For this review, take the finished solid that the model builds, in its own axes (mm). Face numbers are marked on the shaded views. Coordinates: 2 decimals unless noted, no trailing zeros. Loops run counter-clockwise (first coordinate to the right, second up) from the corner with the lowest first, then second, coordinate; pieces in that order, holes last. Notation, with made-up numbers: (52, 29) -> (87, 29) arc R4 ccw to (87, 34) -> close; hole circle Ø3 at (-25.5, 74). An arc over 180 degrees is marked (long way). Answer in a Markdown table with one row per item.
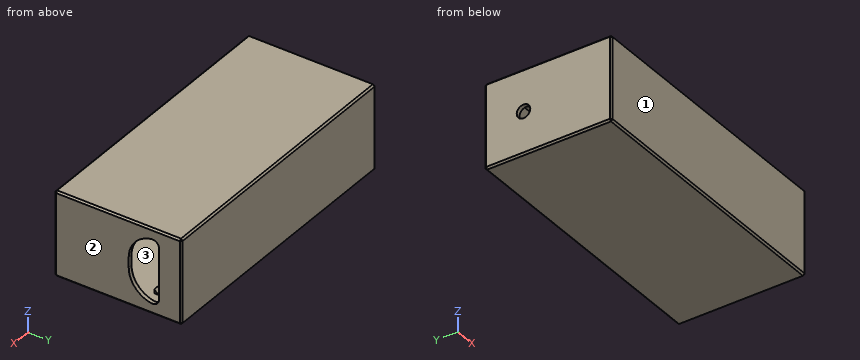
from build123d import *

# Parameters (mm, degrees)
SKETCH1_W           = 82.5
SKETCH1_H           = 25
SKETCH1_W_2         = 80.1
SKETCH1_H_2         = 22.6
BOSS_EXTRUDE1_DEPTH = 23.2
SKETCH1_2_W         = 82.5
SKETCH1_2_H         = 25
SKETCH1_2_W_2       = 80.1
SKETCH1_2_H_2       = 22.6
BOSS_EXTRUDE2_DEPTH = 2
SKETCH2_W           = 2.5
SKETCH2_H           = 5.55
BOSS_EXTRUDE3_DEPTH = 5
SKETCH8_W           = 82.5
SKETCH8_H           = 25
SKETCH8_W_2         = 80.1
SKETCH8_H_2         = 22.6
BOSS_EXTRUDE4_DEPTH = 11.2
SKETCH10_W          = 82.5
SKETCH10_H          = 25
BOSS_EXTRUDE6_DEPTH = 1.2
SKETCH11_W          = 19
SKETCH11_H          = 9
CUT_EXTRUDE1_DEPTH  = 1.2
FILLET1_R           = 8
FILLET2_R           = 2
CHAMFER1_SIZE       = 0.5
CHAMFER2_SIZE       = 2
SKETCH12_R          = 2
CUT_EXTRUDE2_DEPTH  = 1.2


with BuildPart() as part:
    # Sketch1 → Boss-Extrude1 (new body)
    with BuildSketch(Plane(origin=(0, 0, 0), x_dir=(1, 0, 0), z_dir=(0, 1, 0))):
        Rectangle(SKETCH1_W, SKETCH1_H)
        Rectangle(SKETCH1_W_2, SKETCH1_H_2, mode=Mode.SUBTRACT)
    extrude(amount=BOSS_EXTRUDE1_DEPTH)

    # Sketch1_2 → Boss-Extrude2 (add)
    # profile 1 of 2: a face of its own
    with BuildSketch(Plane(origin=(0, 0, 0), x_dir=(1, 0, 0), z_dir=(0, 1, 0))):
        Rectangle(SKETCH1_2_W, SKETCH1_2_H)
        Rectangle(SKETCH1_2_W_2, SKETCH1_2_H_2, mode=Mode.SUBTRACT)
    # profile 2 of 2: a face of its own
    with BuildSketch(Plane(origin=(0, 0, 0), x_dir=(1, 0, 0), z_dir=(0, 1, 0))):
        Rectangle(SKETCH1_2_W_2, SKETCH1_2_H_2)
    extrude(amount=-BOSS_EXTRUDE2_DEPTH)

    # Sketch2 → Boss-Extrude3 (add)
    with BuildSketch(Plane(origin=(0, 0, 0), x_dir=(1, 0, 0), z_dir=(0, 1, 0))):
        with Locations((-38.8, 8.525)):
            Rectangle(SKETCH2_W, SKETCH2_H)
        with Locations((-38.8, -8.525)):
            Rectangle(SKETCH2_W, SKETCH2_H)
        with Locations((38.8, -8.525)):
            Rectangle(SKETCH2_W, SKETCH2_H)
        with Locations((38.8, 8.525)):
            Rectangle(SKETCH2_W, SKETCH2_H)
    extrude(amount=BOSS_EXTRUDE3_DEPTH)

    # Sweep2: sweep along a path in Sketch3
    with BuildLine(Plane(origin=(0, 23.2, 0), x_dir=(1, 0, 0), z_dir=(0, 1, 0))) as sweep2_path:
        Line((-35, 11.3), (35, 11.3))
    # Sketch4 → Sweep2 (sweep)
    with BuildSketch(Plane(origin=(0, 0, 0), x_dir=(0, 0, -1), z_dir=(1, 0, 0))):
        Polygon((10.1, 23.2), (11.3, 24.4), (12.5, 24.4), (12.5, 23.2), align=None)
    sweep2 = sweep(path=sweep2_path.line)

    # Mirror1: Sweep2 across plane
    add(sweep2.mirror(Plane.XY))

    # Sketch8 → Boss-Extrude4 (add)
    with BuildSketch(Plane(origin=(0, 23.2, 0), x_dir=(1, 0, 0), z_dir=(0, 1, 0))):
        Rectangle(SKETCH8_W, SKETCH8_H)
        Rectangle(SKETCH8_W_2, SKETCH8_H_2, mode=Mode.SUBTRACT)
    extrude(amount=BOSS_EXTRUDE4_DEPTH)

    # Sketch10 → Boss-Extrude6 (add)
    with BuildSketch(Plane(origin=(0, 34.4, 0), x_dir=(1, 0, 0), z_dir=(0, 1, 0))):
        Rectangle(SKETCH10_W, SKETCH10_H)
    extrude(amount=BOSS_EXTRUDE6_DEPTH)

    # Sketch11 → Cut-Extrude1 (cut)
    with BuildSketch(Plane(origin=(41.25, 0, 0), x_dir=(0, 0, -1), z_dir=(1, 0, 0))):
        with Locations((0, 24.5)):
            Rectangle(SKETCH11_W, SKETCH11_H)
    extrude(amount=-CUT_EXTRUDE1_DEPTH, mode=Mode.SUBTRACT)

    # Fillet1
    fillet1_edges = [part.edges().sort_by_distance(p)[0] for p in [
        (40.65, 20, -9.5),
        (40.65, 20, 9.5),
    ]]
    fillet(fillet1_edges, radius=FILLET1_R)

    # Fillet2
    fillet2_edges = [part.edges().sort_by_distance(p)[0] for p in [
        (40.65, 29, 9.5),
        (40.65, 29, -9.5),
    ]]
    fillet(fillet2_edges, radius=FILLET2_R)

    # Chamfer1
    chamfer1_edges = [part.edges().sort_by_distance(p)[0] for p in [
        (0, 35.6, -12.5),
        (-41.25, 35.6, 0),
        (0, 35.6, 12.5),
        (41.25, 35.6, 0),
        (41.25, -2, 0),
        (0, -2, 12.5),
        (-41.25, -2, 0),
        (0, -2, -12.5),
        (-41.25, 16.8, -12.5),
        (41.25, 16.8, -12.5),
        (41.25, 16.8, 12.5),
        (-41.25, 16.8, 12.5),
    ]]
    chamfer(chamfer1_edges, length=CHAMFER1_SIZE)

    # Chamfer2
    chamfer2_edges = [part.edges().sort_by_distance(p)[0] for p in [
        (0, 34.4, -11.3),
        (-40.05, 34.4, 0),
        (0, 34.4, 11.3),
        (40.05, 34.4, 0),
    ]]
    chamfer(chamfer2_edges, length=CHAMFER2_SIZE)

    # Sketch12 → Cut-Extrude2 (cut)
    with BuildSketch(Plane.ZY.offset(41.25)):
        with Locations((0, 24)):
            Circle(SKETCH12_R)
    extrude(amount=-CUT_EXTRUDE2_DEPTH, mode=Mode.SUBTRACT)


solid = part.part
Item 1: Take a section at A-A, the plane z = 0. State the section outline as (x, y) points, and give its area (3 significant figures).
Worked answers:
| item | result |
|---|---|
| outline | (-41.25, -1.5) -> (-40.75, -2) -> (40.75, -2) -> (41.25, -1.5) -> (41.25, 20) -> (40.05, 20) -> (40.05, 0) -> (-40.05, 0) -> (-40.05, 22) -> (-41.25, 22) -> close; (-41.25, 26) -> (-40.05, 26) -> (-40.05, 32.4) -> (-38.05, 34.4) -> (38.05, 34.4) -> (40.05, 32.4) -> (40.05, 29) -> (41.25, 29) -> (41.25, 35.1) -> (40.75, 35.6) -> (-40.75, 35.6) -> (-41.25, 35.1) -> close |
| area | 334 mm² |
Item 2: Insertion check: pin 1 (1.3 mm diameter, centred on x = 41, z = 3.5, fed in from -Y). The pin has a flat end and moves straight along its axis. Give the tip position at first contact, or say it passes through.
Worked answers:
| item | result |
|---|---|
| pin 1 | y = -2 |
Item 3: The part is to be moulded in two halves that separate along X. For the marked faces 1, 2 and 3, say which applies: +X half, -X half, draft (parallel to the pull), parting line (faces both ways), or undercut.
Worked answers:
| item | result |
|---|---|
| face 1 | draft |
| face 2 | +X half |
| face 3 | undercut |
Item 4: Take a section at C-C, the plane y = 4. State the section outline as (x, z) points, and give its area (3 significant figures).
Worked answers:
| item | result |
|---|---|
| outline | (-41.25, -12) -> (-40.75, -12.5) -> (40.75, -12.5) -> (41.25, -12) -> (41.25, 12) -> (40.75, 12.5) -> (-40.75, 12.5) -> (-41.25, 12) -> close; hole (-40.05, -5.75) -> (-37.55, -5.75) -> (-37.55, -11.3) -> (37.55, -11.3) -> (37.55, -5.75) -> (40.05, -5.75) -> (40.05, 5.75) -> (37.55, 5.75) -> (37.55, 11.3) -> (-37.55, 11.3) -> (-37.55, 5.75) -> (-40.05, 5.75) -> close |
| area | 307 mm² |
Item 5: Take a section at B-B, the plane x = 23.5. State the section outline as (y, z) points, and give its area (4 significant figures).
Worked answers:
| item | result |
|---|---|
| outline | (-2, -12) -> (-1.5, -12.5) -> (35.1, -12.5) -> (35.6, -12) -> (35.6, 12) -> (35.1, 12.5) -> (-1.5, 12.5) -> (-2, 12) -> close; hole (0, -11.3) -> (23.2, -11.3) -> (23.2, -10.1) -> (24.4, -11.3) -> (32.4, -11.3) -> (34.4, -9.3) -> (34.4, 9.3) -> (32.4, 11.3) -> (24.4, 11.3) -> (23.2, 10.1) -> (23.2, 11.3) -> (0, 11.3) -> close |
| area | 167.5 mm² |
Item 6: For L1, parallel to X at y = 17.5, z = -3; L2, parallel to Y at x = 30, z = -8.25; L3, parallel to X at y = 1.5, z = 7.75, list the stretches that pass through material, from the lowest coordinate up.
Worked answers:
| item | result |
|---|---|
| L1 | -41.25 to -40.05, 40.05 to 41.25 |
| L2 | -2 to 0, 34.4 to 35.6 |
| L3 | -41.25 to -37.55, 37.55 to 41.25 |
